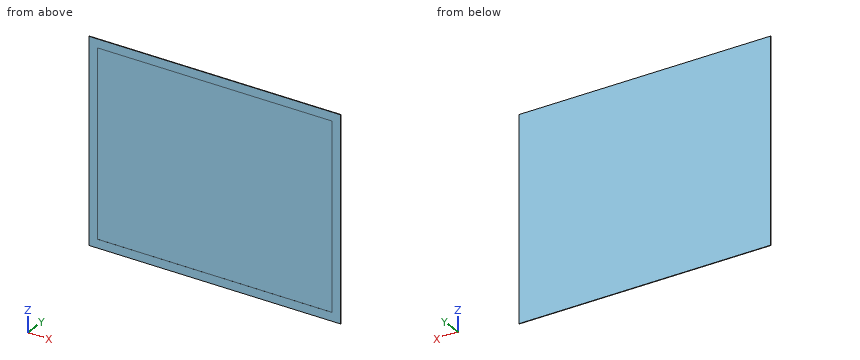
```python
from build123d import *

# Parameters (mm, degrees)
F0_W     = 508
F0_H     = 406.4
F1_DEPTH = 0.635
F2_W     = 473.456
F2_H     = 371.856
F3_DEPTH = 0.0762


with BuildPart() as f1:
    # F0 (on Front) → F1 (new body, symmetric)
    with BuildSketch(Plane.XZ):
        Rectangle(F0_W, F0_H)
    extrude(amount=F1_DEPTH, both=True)

    # F2 (on face) → F3 (cut)
    with BuildSketch(Plane.XZ.offset(0.635)):
        Rectangle(F2_W, F2_H)
    extrude(amount=-F3_DEPTH, mode=Mode.SUBTRACT)


solid = f1.part
```
Here's how the part is built. I have some questions about the finished solid (model axes, mm). Give positions to 0.01 mm unless a question says otherwise; leave off trailing zeros. Loops run counter-clockwise (first coordinate to the right, second up) from the corner with the lowest first, then second, coordinate; pieces in that order, holes last. Notation, with made-up numbers: M 23,-21.5 L 39,-21.5 A15 cw 39,-12.5 Z; hole C 50.5,57.5 d9. An arc over 180 degrees is marked long. Use one line per item in the form item = value. Start each with the question number.
Q1. I need wall thicknesses on line 1 along X through (y, z) = (-0.6, 117); line 2 along Y through (x, z) = (98, 175) (3 decimals). Which ranges of each line are inside material? Lowest first, please.
Q2. If we section it at B-B (x = -203): Write out the boundary of the cut face in (y, z) (3 decimals), then the cut area to 3 significant figures.
Q3. If we section it at A-A (z = -55): Write out the boundary of the cut face in (x, y) (3 decimals).
Q4. Will this pin go through, and if not, where does the flat tip stop? pin 1 Ø6 at (x, z) = (94, 10) entering from -Y.
Taken from the geometry:
q1.line_1 = -254 to -236.73, 236.73 to 254
q1.line_2 = -0.559 to 0.635
q2.outline = M -0.635,-203.2 L 0.635,-203.2 L 0.635,203.2 L -0.635,203.2 L -0.635,185.928 L -0.559,185.928 L -0.559,-185.928 L -0.635,-185.928 Z
q2.area = 488 mm^2
q3.outline = M -254,-0.635 L -236.728,-0.635 L -236.728,-0.559 L 236.728,-0.559 L 236.728,-0.635 L 254,-0.635 L 254,0.635 L -254,0.635 Z
q4.pin_1 = -0.56
